Input: part model. Units: mm. Frame: model coordinates. A direction names the side the tool comes from. Coordinates: 2 decimals unless noted, no trailing zeros. Write each loop counter-clockwise with the first axis right and the second up, starting at its lowest first coordinate (ties: lowest second). Pieces come first, ordered by that corner, then holes. Notation, with made-up numbers: (23.25, 59.5) -> (53.25, 59.5) arc R13 ccw to (53.25, 70.5) -> close; hole circle Ø11 at (-31, -37.75). An arc over 180 degrees is marked (long way). Use one line per item in the form item = value. Start each with the question number.
(1) Cut plane C-C on y = 11. Return the cut outline in (x, z), plus the area to 3 significant figures.
(2) Cut plane D-D on x = 4.25. Return the cut outline in (y, z).
(3) Ray query, line 1 along X through (y, z) = (15, 4.7); line 2 along Z through (x, y) = (9, 16.5); line 3 along Y through (x, z) = (0, -5.65). Return the intervals inside material, ascending.
(4) First-contact query: pin 1 (3 mm diameter, centred on x = 2.5, z = -5, fed in from -Y); pin 2 (1.5 mm diameter, centred on x = 14, z = 6, fed in from +Y); pin 3 (1.5 mm diameter, centred on x = 14.5, z = 5.5, fed in from -Y). Flat tips, straight axial feed; report the tip coordinate or a pass-through.
(5) Cut plane A-A on x = 0. Return the cut outline in (y, z).
(6) Pull-direction query (Y, two-part tool) for faces 1 (the face through (0, 30, -5)), 2 (the face through (0, -32.5, -5)), 3 (the face through (-1, 30, -3)); classes: released by +Y, released by -Y, zero draft, split by the parting line, or undercut.
(7) Cut plane B-B on y = 27.5. Return the cut outline in (x, z).
(8) Set-up query: faces 4 (the face through (10, 15, 4)), 5 (the face through (0, -32.5, 5)), 6 (the face through (-1, 30, 3)), 7 (the face through (-1, -35, -3)), 8 (the face through (11, 20, -5)). Return all of +Z, -Z, +X, -X, +Y, -Y with unobstructed straight access to the full face (end or side cutting, diameter ignored); none if empty.
```python
from build123d import *

# Parameters (mm, degrees)
SKETCH_1_W                = 10
SKETCH_1_H                = 14
EXTRUDE_1_DEPTH           = 32.5
SKETCH_7_W                = 13
SKETCH_7_H                = 10
EXTRUDE_3_DEPTH           = 7
SKETCH_8_W                = 13
SKETCH_8_H                = 10
CUT_EXTRUDE_3_DEPTH       = 4
SKETCH_10_R               = 2.5
CUT_EXTRUDE_4_DEPTH       = 8
CUT_EXTRUDE_4_DEPTH_BACK  = 8
SKETCH_14_W               = 10
SKETCH_14_H               = 10
CUT_EXTRUDE_8_DEPTH       = 3
SKETCH_15_W               = 10
SKETCH_15_H               = 10
EXTRUDE_4_DEPTH           = 3
SKETCH_16_R               = 2.5
CUT_EXTRUDE_9_DEPTH       = 8
CUT_EXTRUDE_9_DEPTH_BACK  = 8
SKETCH_17_R               = 2.5
CUT_EXTRUDE_10_DEPTH      = 8
CUT_EXTRUDE_10_DEPTH_BACK = 8


with BuildPart() as part:
    # 草图1 → 凸台-拉伸1 (new body, symmetric)
    with BuildSketch(Plane(origin=(0, 0, 0), x_dir=(1, 0, 0), z_dir=(0, 1, 0))):
        Rectangle(SKETCH_1_W, SKETCH_1_H)
    extrude(amount=EXTRUDE_1_DEPTH, both=True)

    # 草图7 → 凸台-拉伸3 (add, symmetric)
    with BuildSketch(Plane.XY):
        with Locations((11.5, 15)):
            Rectangle(SKETCH_7_W, SKETCH_7_H)
    extrude(amount=EXTRUDE_3_DEPTH, both=True)

    # 草图8 → 切除-拉伸3 (cut, symmetric)
    with BuildSketch(Plane.XY):
        with Locations((11.5, 15)):
            Rectangle(SKETCH_8_W, SKETCH_8_H)
    extrude(amount=CUT_EXTRUDE_3_DEPTH, both=True, mode=Mode.SUBTRACT)

    # 草图10 → 切除-拉伸4 (cut, two sides)
    with BuildSketch(Plane.XY) as cut_extrude_4_sk:
        with Locations((13.005535268, 15)):
            Circle(SKETCH_10_R)
    extrude(amount=CUT_EXTRUDE_4_DEPTH, mode=Mode.SUBTRACT)
    extrude(cut_extrude_4_sk.sketch, amount=-CUT_EXTRUDE_4_DEPTH_BACK, mode=Mode.SUBTRACT)

    # 草图14 → 切除-拉伸8 (cut, symmetric)
    with BuildSketch(Plane.XY):
        with Locations((0, 27.5)):
            Rectangle(SKETCH_14_W, SKETCH_14_H)
    extrude(amount=CUT_EXTRUDE_8_DEPTH, both=True, mode=Mode.SUBTRACT)

    # 草图15 → 凸台-拉伸4 (add, symmetric)
    with BuildSketch(Plane.XY):
        with Locations((0, -37.5)):
            Rectangle(SKETCH_15_W, SKETCH_15_H)
    extrude(amount=EXTRUDE_4_DEPTH, both=True)

    # 草图16 → 切除-拉伸9 (cut, two sides)
    with BuildSketch(Plane.XY) as cut_extrude_9_sk:
        with Locations((0, 27.5)):
            Circle(SKETCH_16_R)
    extrude(amount=CUT_EXTRUDE_9_DEPTH, mode=Mode.SUBTRACT)
    extrude(cut_extrude_9_sk.sketch, amount=-CUT_EXTRUDE_9_DEPTH_BACK, mode=Mode.SUBTRACT)

    # 草图17 → 切除-拉伸10 (cut, two sides)
    with BuildSketch(Plane.XY) as cut_extrude_10_sk:
        with Locations((0, -37.5)):
            Circle(SKETCH_17_R)
    extrude(amount=CUT_EXTRUDE_10_DEPTH, mode=Mode.SUBTRACT)
    extrude(cut_extrude_10_sk.sketch, amount=-CUT_EXTRUDE_10_DEPTH_BACK, mode=Mode.SUBTRACT)


solid = part.part
```
Values:
q1.outline = (-5, -7) -> (18, -7) -> (18, -4) -> (5, -4) -> (5, 4) -> (18, 4) -> (18, 7) -> (-5, 7) -> close
q1.area = 218 mm2
q2.outline = (-42.5, -3) -> (-32.5, -3) -> (-32.5, -7) -> (32.5, -7) -> (32.5, -3) -> (22.5, -3) -> (22.5, 3) -> (32.5, 3) -> (32.5, 7) -> (-32.5, 7) -> (-32.5, 3) -> (-42.5, 3) -> close
q3.line_1 = -5 to 10.51, 15.51 to 18
q3.line_2 = -7 to -4, 4 to 7
q3.line_3 = -32.5 to 25, 30 to 32.5
q4.pin_1 = -32.5
q4.pin_2 = 20
q4.pin_3 = 10
q5.outline = (-42.5, -3) -> (-40, -3) -> (-40, 3) -> (-42.5, 3) -> close; (-35, -3) -> (-32.5, -3) -> (-32.5, -7) -> (25, -7) -> (25, -3) -> (22.5, -3) -> (22.5, 3) -> (25, 3) -> (25, 7) -> (-32.5, 7) -> (-32.5, 3) -> (-35, 3) -> close; (30, -7) -> (32.5, -7) -> (32.5, -3) -> (30, -3) -> close; (30, 3) -> (32.5, 3) -> (32.5, 7) -> (30, 7) -> close
q6.face_1 = undercut
q6.face_2 = released by -Y
q6.face_3 = zero draft
q7.outline = (-5, -7) -> (-2.5, -7) -> (-2.5, -3) -> (-5, -3) -> close; (-5, 3) -> (-2.5, 3) -> (-2.5, 7) -> (-5, 7) -> close; (2.5, -7) -> (5, -7) -> (5, -3) -> (2.5, -3) -> close; (2.5, 3) -> (5, 3) -> (5, 7) -> (2.5, 7) -> close
q8.face_4 = +X, +Y, -Y
q8.face_5 = +Z, +X, -X, -Y
q8.face_6 = +X, -X, +Y
q8.face_7 = -Z, +X, -X, -Y
q8.face_8 = +Z, -Z, +X, +Y
